Verification items for the finished model (mm, model axes). Give positions to 0.01 mm unless a question says otherwise; leave off trailing zeros. Loops run counter-clockwise (first coordinate to the right, second up) from the corner with the lowest first, then second, coordinate; pieces in that order, holes last. Notation, with made-up numbers: M -5.75,77.25 L 45.25,77.25 A14 cw 45.25,99.25 Z; hole C -4.75,15.25 d1. An arc over 180 degrees is marked long. Use a Markdown table: item, result.
from build123d import *

# Parameters (mm, degrees)
SKETCH_1_W          = 179.63
SKETCH_1_H          = 220
EXTRUDE_1_DEPTH     = 5
SKETCH_2_W          = 179.63
SKETCH_2_H          = 220
EXTRUDE_2_DEPTH     = 103
CUT_EXTRUDE_1_DEPTH = 375


with BuildPart() as part:
    # Эскиз1 → Бобышка-Вытянуть1 (new body)
    with BuildSketch(Plane(origin=(0, 0, 0), x_dir=(1, 0, 0), z_dir=(0, 1, 0))):
        with Locations((-85.713003719, 94.130447377)):
            Rectangle(SKETCH_1_W, SKETCH_1_H)
    extrude(amount=EXTRUDE_1_DEPTH)

    # Эскиз2 → Бобышка-Вытянуть2 (add)
    with BuildSketch(Plane(origin=(0, 5, 0), x_dir=(1, 0, 0), z_dir=(0, 1, 0))):
        with Locations((-85.713003719, 94.130447377)):
            Rectangle(SKETCH_2_W, SKETCH_2_H)
    extrude(amount=EXTRUDE_2_DEPTH)

    # Эскиз3 → Вырез-Вытянуть1 (cut)
    with BuildSketch(Plane(origin=(4.101996281, 0, 0), x_dir=(0, 0, -1), z_dir=(1, 0, 0))):
        Polygon((-5.789329855, 66.247834785), (204.130447377, 10), (204.130447377, 108), (-15.869552623, 108), (-15.869552623, 68.948822335), align=None)
    extrude(amount=-CUT_EXTRUDE_1_DEPTH, mode=Mode.SUBTRACT)


solid = part.part
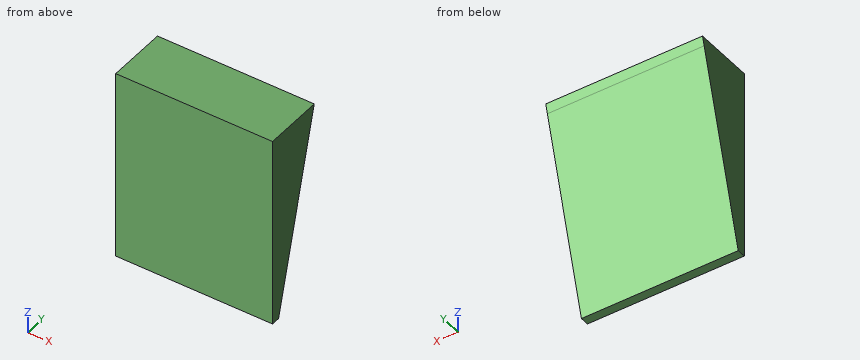
(1) Cross-section at A-A on x = -38. Record the cut outline in (y, z), then the cut area to 3 significant figures.
Results below:
| item | result |
|---|---|
| outline | M 0,-204.13 L 10,-204.13 L 68.95,15.87 L 0,15.87 Z |
| area | 8,680 mm^2 |
(2) Cross-section at B-B on z = -64. Record the cut outline in (x, y), then the cut area to 3 significant figures.
Results below:
| item | result |
|---|---|
| outline | M -175.53,0 L 4.1,0 L 4.1,47.55 L -175.53,47.55 Z |
| area | 8,540 mm^2 |
(3) Gauge pin test, flat ends, axial feed: P1, Ø1.5, axis at x = -104.5, z = -147.5, coming from the +Y side; P2, Ø10, axis at x = -62.5, z = -118.5, coming from the +Y side; P3, Ø8, axis at x = -76, z = -177.5, coming from the -Y side. Record the tip position at first contact, or that the pin passes through.
Results below:
| item | result |
|---|---|
| P1 | y = 25.38 |
| P2 | y = 34.28 |
| P3 | y = 0 |
(4) Material ranges on line 1 (Y direction, x = -97, z = -125); line 2 (Y direction, x = -74, z = -68), recorded low to high.
Results below:
| item | result |
|---|---|
| line 1 | 0 to 31.2 |
| line 2 | 0 to 46.48 |
(5) Cross-section at C-C on y = 49. Record the cut outline in (x, z), then the cut area to 3 significant figures.
Results below:
| item | result |
|---|---|
| outline | M -175.53,-58.58 L 4.1,-58.58 L 4.1,15.87 L -175.53,15.87 Z |
| area | 13,400 mm^2 |
